Model file for the job. Use its own axes, mm. Face numbers are marked on the shaded views. A direction names the side the tool comes from. Round coordinates to 2 decimals unless told otherwise and drop trailing zeros. Write each loop counter-clockwise with the first axis right and the second up, starting at its lowest first coordinate (ties: lowest second). Pieces come first, ordered by that corner, then holes. Notation, with made-up numbers: (60.25, 84.5) - (80.25, 84.5) arc R27 cw to (80.25, 110.5) - close; hole circle Ø1 at (79, -5.75). An arc over 180 degrees is marked (long way). One line per item, written item: value.
from build123d import *

# Parameters (mm, degrees)
F1_DEPTH  = 8.5
F3_DEPTH  = 1
F5_W      = 21.3351653656
F5_H      = 16.6395662818
F6_DEPTH  = 25.4
F8_W      = 32.5405728072
F8_H      = 36.5617219359
F9_DEPTH  = 25.4
F12_W     = 39.0807809308
F12_H     = 30.5973365903
F13_DEPTH = 25.4
F15_W     = 34.2101305723
F15_H     = 32.0557234809
F16_DEPTH = 25.4
F18_W     = 10.4850952048
F18_H     = 24.5708920993
F19_DEPTH = 25.4
F23_T     = -1


with BuildPart() as f1:
    # F0 (on Top) → F1 (new body)
    with BuildSketch(Plane.XY):
        Polygon((12, -12), (12, 0), (2.0081724885, -9.9918275115), (3.148298335, -11.131953358), align=None)
    extrude(amount=F1_DEPTH)

    # F2 (on face) → F3 (cut)
    with BuildSketch(Plane.XY.offset(8.5)):
        Polygon((12, -6), (12, 0), (7.0040862443, -4.9959137557), align=None)
    extrude(amount=-F3_DEPTH, mode=Mode.SUBTRACT)

    # F5 (on face) → F6 (cut)
    with BuildSketch(Plane(origin=(-0.2736218822, -1.3614281972, 7.8754394827), x_dir=(0.999414466, -0.0058284524, 0.033715788), z_dir=(-0.0342158621, -0.170243838, 0.984807753))):
        with Locations((9.1339054634, -6.3430479495)):
            Rectangle(F5_W, F5_H)
    extrude(amount=F6_DEPTH, mode=Mode.SUBTRACT)

    # F8 (on 3pt) → F9 (cut)
    with BuildSketch(Plane(origin=(-2.047796356, -1.8446305737, 2.5928305655), x_dir=(0.8409146633, -0.3137144476, 0.44096006), z_dir=(-0.5411677458, -0.4874774616, 0.6852030322))):
        with Locations((12.2363092378, -5.4249586537)):
            Rectangle(F8_W, F8_H)
    extrude(amount=F9_DEPTH, mode=Mode.SUBTRACT)

    # F12 (on 3pt) → F13 (cut)
    with BuildSketch(Plane(origin=(-2.1635826482, -3.1806122044, 3.7144904348), x_dir=(0.9144921522, -0.2631581438, 0.3073302701), z_dir=(-0.4046036376, -0.5947945963, 0.6946332016))):
        with Locations((12.1668963693, -3.5860668868)):
            Rectangle(F12_W, F12_H)
    extrude(amount=F13_DEPTH, mode=Mode.SUBTRACT)

    # F15 (on 3pt) → F16 (cut)
    with BuildSketch(Plane(origin=(-0.8887297085, -9.0626123757, 3.8943302941), x_dir=(0.995965621, -0.0824459089, 0.0354281511), z_dir=(-0.0897356216, -0.9150579155, 0.393213084))):
        with Locations((12.4972742051, -3.3018724062)):
            Rectangle(F15_W, F15_H)
    extrude(amount=F16_DEPTH, mode=Mode.SUBTRACT)

    # F18 (on 3pt) → F19 (cut)
    with BuildSketch(Plane(origin=(-2.1149465474, -2.1149465474, 2.8176241463), x_dir=(0.8573741534, -0.3089777782, 0.4116336886), z_dir=(0.5146936574, 0.5146936574, -0.6856973662))):
        with Locations((7.849192596, 5.699301837)):
            Rectangle(F18_W, F18_H)
    extrude(amount=-F19_DEPTH, mode=Mode.SUBTRACT)

    # F20: F1 across face


with BuildPart() as f1_1:
    add(f1.part)
    add(f1.part.mirror(Plane(origin=(8.1142893011, -3.8857106989, 3.3333333333), x_dir=(-0.7071067812, -0.7071067812, 0), z_dir=(-0.7071067812, 0.7071067812, 0))))

    # F21: F1 across face


with BuildPart() as f1_2:
    add(f1_1.part)
    add(f1_1.part.mirror(Plane(origin=(12, -5.2108536925, 3.5209267252), x_dir=(0, 1, 0), z_dir=(1, 0, 0))))

    # F22: F1 across face


with BuildPart() as f1_3:
    add(f1_2.part)
    add(f1_2.part.mirror(Plane(origin=(12, 0, 3.5209267252), x_dir=(-1, 0, 0), z_dir=(0, 1, 0))))

    # F23
    f23_openings = [f1_3.faces().sort_by_distance(p)[0] for p in [
        (12, 0, 0),
    ]]
    offset(amount=F23_T, openings=f23_openings)


solid = f1_3.part
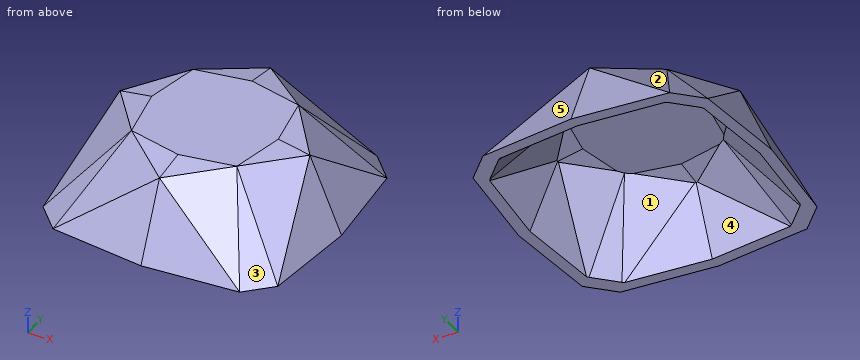
1. Band-saw the part on B-B on y = 2.5. Write the cut outline in (x, z), plus the area to 3 significant figures.
Report:
outline: (0.25, 0) - (1.34, 0) - (3.15, 4.21) - (5.62, 6.33) - (6.59, 6.5) - (17.41, 6.5) - (18.38, 6.33) - (20.85, 4.21) - (22.66, 0) - (23.75, 0) - (21.6, 5.01) - (19, 7.24) - (17.5, 7.5) - (6.5, 7.5) - (5, 7.24) - (2.4, 5.01) - close
area: 30.8 mm²
2. Band-saw the part on C-C on x = 14. Write the cut outline in (y, z), plus the area to 3 significant figures.
Report:
outline: (-11.8, 0) - (-10.71, 0) - (-8.73, 4.61) - (-6.78, 6.28) - (-5.51, 6.5) - (5.51, 6.5) - (6.78, 6.28) - (8.73, 4.61) - (10.71, 0) - (11.8, 0) - (9.48, 5.4) - (7.4, 7.19) - (5.6, 7.5) - (-5.6, 7.5) - (-7.4, 7.19) - (-9.48, 5.4) - close
area: 31.0 mm²
3. Mould opens along X. For the marked faces 1, 2 and 3 say: released by +X, released by -X, zero draft, split by the parting line, or undercut.
Report:
face 1: undercut
face 2: released by -X
face 3: released by +X
4. Wall check: probe 1 along Z at (x, y) = (8.5, -2.25); probe 2 along Y at (x, z) = (7, 6); probe 3 along Y at (x, z) = (15.75, 4.5). Give the ranges that are in metal, low to high. Write a range as [from, to].
Report:
probe 1: [6.5, 7.5]
probe 2: [-6.74, -5.05], [5.05, 6.74]
probe 3: [-9.35, -7.67], [7.67, 9.35]
5. Band-saw the part on A-A on x = 5.25. Write the cut outline in (y, z), plus the area to 3 significant figures.
Report:
outline: (-11.34, 0) - (-10.25, 0) - (-9.88, 0.86) - (-7.96, 2.5) - (-5.99, 3.98) - (-2.03, 6.28) - (0, 6.35) - (2.03, 6.28) - (5.99, 3.98) - (7.96, 2.5) - (9.88, 0.86) - (10.25, 0) - (11.34, 0) - (10.63, 1.66) - (7.79, 4.09) - (6.1, 5.36) - (2.81, 7.27) - (0, 7.37) - (-2.81, 7.27) - (-6.1, 5.36) - (-7.79, 4.09) - (-10.63, 1.66) - close
area: 30.3 mm²
6. Drop flat-ended pins along their axis: pin 1 (9.5 mm diameter, centred on x = 12, y = -1, fed in from -Z); pin 2 (1 mm diameter, centred on y = -6, z = 4, fed in from +X); pin 3 (3 mm diameter, centred on y = 4.5, z = 3, fed in from -X). Give the stop position or say it passes through.
Report:
pin 1: z = 6.5
pin 2: x = 21.08
pin 3: x = 1.07
7. Tool access for the marked faces 4 and 5: list every direction of +Z, -Z, +X, -X, +Y, -Y with a clear straight run to the whole face (end or side of a thin tool).
Report:
face 4: -Z
face 5: +Z, +X, +Y
8. Band-saw the part on D-D on x = 19.25. Write the cut outline in (y, z).
Report:
outline: (-11.29, 0) - (-10.2, 0) - (-10, 0.47) - (-8.76, 1.52) - (-6.3, 3.37) - (-1.41, 6.22) - (0, 6.27) - (1.41, 6.22) - (6.3, 3.37) - (8.76, 1.52) - (10, 0.47) - (10.2, 0) - (11.29, 0) - (10.75, 1.26) - (8.58, 3.12) - (6.41, 4.74) - (2.18, 7.21) - (0, 7.28) - (-2.18, 7.21) - (-6.41, 4.74) - (-8.58, 3.12) - (-10.75, 1.26) - close
